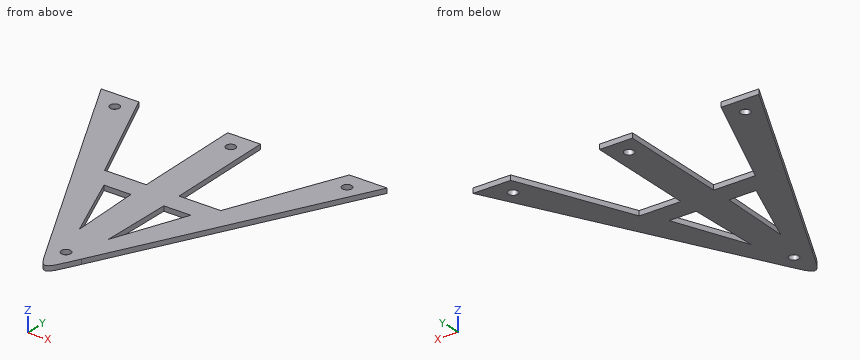
```python
from build123d import *

# Parameters (mm, degrees)
F1_DEPTH   = 3
F4_D       = 5.8
F4_ON_F2_D = 5.8


with BuildPart() as f1:
    # F0 (on Top) → F1 (new body)
    with BuildSketch(Plane.XY):
        with BuildLine():
            add(Edge.make_bspline(
                [(10.4103045447, -67.024596429), (8.982228674, -69.7149249082), (6.3151262234, -75.1432740364), (-0.0293251038, -86.7211019833), (-6.4479244726, -74.8137621783), (-9.3542937571, -69.1019658828), (-10.9111016264, -66.0546038255)],
                knots=[0, 0, 0, 0, 0.2518062745, 0.4931803978, 0.7376570715, 1, 1, 1, 1], degree=3))
            Line((10.4103045447, -67.024596429), (87.4111636015, 82.118173113))
            Line((87.4111636015, 82.118173113), (64.3657235353, 82.118173113))
            Line((64.3657235353, 82.118173113), (35.5318893309, 14.5721204152))
            Line((35.5318893309, 14.5721204152), (10.0382260192, 14.5721204152))
            Line((10.0382260192, 14.5721204152), (10.0382260192, 82.118173113))
            Line((10.0382260192, 82.118173113), (0, 82.118173113))
            Line((0, 82.118173113), (-10.0382260192, 82.118173113))
            Line((-10.0382260192, 82.118173113), (-10.0382260192, 14.5721204152))
            Line((-10.0382260192, 14.5721204152), (-35.5318893309, 14.5721204152))
            Line((-35.5318893309, 14.5721204152), (-64.3657235353, 82.118173113))
            Line((-64.3657235353, 82.118173113), (-87.4111636015, 82.118173113))
            Line((-87.4111636015, 82.118173113), (-10.9111016264, -66.0546038255))
        make_face()
        Polygon((-10.0382260192, 1.8761669675), (-8.8880723342, -42.5141826272), (-26.5612563327, 1.8761669675), align=None, mode=Mode.SUBTRACT)
        Polygon((8.8880723342, -42.5141826272), (10.0382260192, 1.8761669675), (26.5612563327, 1.8761669675), align=None, mode=Mode.SUBTRACT)
    extrude(amount=F1_DEPTH)

    # F4 (through all)
    with Locations(Plane(origin=(0, 0, 0), x_dir=(1, 0, 0), z_dir=(0, 0, -1))):
        with Locations((-71.0588246584, -71.1358040571), (0, -71.1358040571), (71.0588246584, -71.1358040571)):
            Hole(F4_D / 2)

    # F4 on F2 (through all)
    with Locations(Plane(origin=(0, 0, 0), x_dir=(1, 0, 0), z_dir=(0, 0, -1))):
        with Locations((0, 65.6056776643)):
            Hole(F4_ON_F2_D / 2)


solid = f1.part
```
Design review of the part built by this model. Coordinates are the model's own, in mm. Coordinates: 2 decimals unless noted, no trailing zeros. Loops run counter-clockwise (first coordinate to the right, second up) from the corner with the lowest first, then second, coordinate; pieces in that order, holes last. Notation, with made-up numbers: (56, 12) - (108, 12) arc R22 ccw to (108, 34) - close; hole circle Ø4 at (-9, 72.25). An arc over 180 degrees is marked (long way). Use CSV: the item, a comma, the result in double quotes. Start each with the question number.
1) Consider section B-B on x = 0. Give the number of separate pieces and of enclosed holes in the cut face, then the cut area to 3 significant figures.
2) For pin 1 Ø1.5 at (x, z) = (19, 1.5) entering from +Y; pin 2 Ø10 at (x, y) = (-68.5, 43.5) entering from -Z, all flat-tipped, find the tip position at first contact; note any pin that passes through.
3) Consider section C-C on x = 21. Write out the cut boundary in (y, z), then the cut area to 3 significant figures.
4) Wall thickness on L1, parallel to Y at x = 0, z = 1.6; L2, parallel to X at y = -27, z = 2.8; L3, parallel to X at y = 1, z = 0.9: over which ranges is each line inside the solid? List them lowest first. Write a range as from..to.
5) Consider section A-A on y = -22. Write out the cut boundary in (x, z).
Geometry says:
1,separate pieces,"3"
1,enclosed holes,"0"
1,area,"460 mm^2"
2,pin 1,"y = 14.57"
2,pin 2,"z = 0"
3,outline,"(-46.51, 0) - (-12.09, 0) - (-12.09, 3) - (-46.51, 3) - close; (1.88, 0) - (14.57, 0) - (14.57, 3) - (1.88, 3) - close"
3,area,"141 mm^2"
4,L1,"-82.88..-68.51, -62.71..68.24, 74.04..82.12"
4,L2,"-31.07..-15.06, -9.29..9.29, 15.06..31.07"
4,L3,"-45.53..-26.21, -10.02..10.02, 26.21..45.53"
5,outline,"(-33.66, 0) - (-17.06, 0) - (-17.06, 3) - (-33.66, 3) - close; (-9.42, 0) - (9.42, 0) - (9.42, 3) - (-9.42, 3) - close; (17.06, 0) - (33.66, 0) - (33.66, 3) - (17.06, 3) - close"
